Build history of the part. All positions in model axes, mm. A direction names the side the tool comes from. Coordinates: 2 decimals unless noted, no trailing zeros. Loops run counter-clockwise (first coordinate to the right, second up) from the corner with the lowest first, then second, coordinate; pieces in that order, holes last. Notation, with made-up numbers: (47.5, 84) - (105.5, 84) arc R32 ccw to (105.5, 122) - close; hole circle Ø8 at (26.25, 79.5). An arc over 180 degrees is marked (long way). One line per item, written item: value.
```python
from build123d import *


with BuildPart() as f3:
    # F3: sweep along a path in F0
    with BuildLine(Plane.XY) as f3_path:
        Line((-23.8125, -254), (-23.8125, 0))
        ThreePointArc((-23.8125, 0), (0, 23.8125), (23.8125, 0))
        Line((23.8125, 0), (23.8125, -152.4))
    # F2 (on offset) → F3 (sweep)
    with BuildSketch(Plane.XZ.offset(254)):
        Polygon((-19.05, 4.7625), (-28.575, 4.7625), (-28.575, -4.7625), (-19.05, -4.7625), (-19.05, 0), align=None)
    sweep(path=f3_path.line)


solid = f3.part
```
Item 1: Pull direction X, two halves, no side cores. Call faces 1 (the face through (-24, -254, 0)), 2 (the face through (-28.575, -125, 0)), 3 (the face through (-0.419, 19.045, 0.067)): released by +X, released by -X, zero draft, split by the parting line, or undercut.
Check result:
face 1: zero draft
face 2: released by -X
face 3: undercut
Item 2: Cut at D-D, the plane x = 15. Write the cut outline in (y, z), then the cut area to 3 significant figures.
Check result:
outline: (11.74, -4.76) - (24.32, -4.76) - (24.32, 4.76) - (11.74, 4.76) - close
area: 120 mm^2
Item 3: Probe probe 1 along X at (y, z) = (-139.5, 1) (3 decimals); probe 2 along X at (y, z) = (-193, 1) (3 decimals). List the from-to ranges inside material, lowest first. Write a range as from..to.
Check result:
probe 1: x = -28.575..-19.05, 19.05..28.575
probe 2: x = -28.575..-19.05
Item 4: Tool access for faces 4 (the face through (-21, -81, -4.762)), 5 (the face through (19.05, -77, 0)), 6 (the face through (24, -152.4, 0)): list every direction of +Z, -Z, +X, -X, +Y, -Y with a clear straight run to the whole face (end or side of a thin tool).
Check result:
face 4: -Z, +X, -X, +Y, -Y
face 5: +Z, -Z, -Y
face 6: +Z, -Z, +X, -Y
Item 5: Drop flat-ended pins along their axis: P1, Ø2, axis at x = -4, z = 1, coming from the -Y side; P2, Ø10, axis at x = -13, y = -222, coming from the +Z side (3 decimals); P3, Ø2, axis at x = -2, z = 0.5, coming from the -Y side; P4, Ø1, axis at x = -7, z = 3, coming from the -Y side. Give the stop position or say it passes through.
Check result:
P1: stops at y = 18.38
P2: passes through
P3: stops at y = 18.81
P4: stops at y = 17.51
Item 6: Cut at B-B, the plane z = -1. Write the cut outline in (x, y) (3 decimals).
Check result:
outline: (-28.575, -254) - (-19.05, -254) - (-19.05, 0) arc R19.05 cw to (19.05, 0) - (19.05, -152.4) - (28.575, -152.4) - (28.575, 0) arc R28.575 ccw to (-28.575, 0) - close
